```python
from build123d import *

# Parameters (mm, degrees)
BOSS_EXTRUDE4_DEPTH = 21
BOSS_EXTRUDE5_START = 3.5
BOSS_EXTRUDE5_DEPTH = 3.5
SKETCH4_W           = 27
SKETCH4_H           = 19
CUT_EXTRUDE4_DEPTH  = 72.268857154
SKETCH3_5_W         = 24.4
SKETCH3_5_H         = 12.66
BOSS_EXTRUDE6_DEPTH = 2
SKETCH5_W           = 51
SKETCH5_H           = 30
BOSS_EXTRUDE7_DEPTH = 10
CUT_EXTRUDE5_DEPTH  = 75.828136419
CUT_EXTRUDE6_REACH  = 76.828
SKETCH8_W           = 24.5
SKETCH8_H           = 19.5
CHAMFER1_SIZE       = 2


with BuildPart() as part:
    # Sketch3 → Boss-Extrude4 (new body)
    with BuildSketch(Plane(origin=(0, 0, 0), x_dir=(1, 0, 0), z_dir=(0, 1, 0))):
        with BuildLine():
            Line((-27, 15), (-27, -39.5))
            ThreePointArc((-27, -39.5), (-26.414213562, -40.914213562), (-25, -41.5))
            Line((-25, -41.5), (25, -41.5))
            ThreePointArc((25, -41.5), (26.414213562, -40.914213562), (27, -39.5))
            Line((27, -39.5), (27, 15))
            ThreePointArc((27, 15), (26.414213562, 16.414213562), (25, 17))
            Line((25, 17), (-25, 17))
            ThreePointArc((-25, 17), (-26.414213562, 16.414213562), (-27, 15))
        make_face()
    extrude(amount=-BOSS_EXTRUDE4_DEPTH)

    # Sketch3<3> → Boss-Extrude5 (add)
    with BuildSketch(Plane(origin=(0, 0, 0), x_dir=(1, 0, 0), z_dir=(0, 1, 0)).offset(BOSS_EXTRUDE5_START)):
        with BuildLine():
            Line((-27, 15), (-27, -39.5))
            ThreePointArc((-27, -39.5), (-26.414213562, -40.914213562), (-25, -41.5))
            Line((-25, -41.5), (25, -41.5))
            ThreePointArc((25, -41.5), (26.414213562, -40.914213562), (27, -39.5))
            Line((27, -39.5), (27, 15))
            ThreePointArc((27, 15), (26.414213562, 16.414213562), (25, 17))
            Line((25, 17), (-25, 17))
            ThreePointArc((-25, 17), (-26.414213562, 16.414213562), (-27, 15))
        make_face()
        Polygon((0, 12), (-1.1, 12), (-1.1, -3.66), (-25.5, -3.66), (-25.5, 15.5), (25.5, 15.5), (25.5, -0.96), (0, -0.96), align=None, mode=Mode.SUBTRACT)
    extrude(amount=-BOSS_EXTRUDE5_DEPTH)

    # Sketch4 → Cut-Extrude4 (cut, through all)
    with BuildSketch(Plane.ZY.offset(27)):
        with Locations((-1.5, -9.5)):
            Rectangle(SKETCH4_W, SKETCH4_H)
    extrude(amount=-CUT_EXTRUDE4_DEPTH, mode=Mode.SUBTRACT)

    # Sketch3<5> → Boss-Extrude6 (add)
    with BuildSketch(Plane(origin=(0, 0, 0), x_dir=(1, 0, 0), z_dir=(0, 1, 0))):
        with Locations((-13.3, 5.67)):
            Rectangle(SKETCH3_5_W, SKETCH3_5_H)
        Polygon((25.5, 12), (0, 12), (0, -0.96), (25.5, -0.96), (25.5, -0.5), align=None)
    extrude(amount=BOSS_EXTRUDE6_DEPTH)

    # Sketch5 → Boss-Extrude7 (add)
    # profile 1 of 2: a face of its own
    with BuildSketch(Plane.XZ.offset(21)):
        with BuildLine():
            ThreePointArc((25, -17), (26.414213562, -16.414213562), (27, -15))
            Line((27, -15), (27, 39.5))
            ThreePointArc((27, 39.5), (26.414213562, 40.914213562), (25, 41.5))
            Line((25, 41.5), (-25, 41.5))
            ThreePointArc((-25, 41.5), (-26.414213562, 40.914213562), (-27, 39.5))
            Line((-27, 39.5), (-27, -15))
            ThreePointArc((-27, -15), (-26.414213562, -16.414213562), (-25, -17))
            Line((-25, -17), (25, -17))
        make_face()
        with Locations((0, -1.5)):
            Rectangle(SKETCH5_W, SKETCH5_H, mode=Mode.SUBTRACT)
    # profile 2 of 2: a face of its own
    with BuildSketch(Plane.XZ.offset(21)):
        with BuildLine():
            ThreePointArc((25, -17), (26.414213562, -16.414213562), (27, -15))
            Line((27, -15), (27, 39.5))
            ThreePointArc((27, 39.5), (26.414213562, 40.914213562), (25, 41.5))
            Line((25, 41.5), (-25, 41.5))
            ThreePointArc((-25, 41.5), (-26.414213562, 40.914213562), (-27, 39.5))
            Line((-27, 39.5), (-27, -15))
            ThreePointArc((-27, -15), (-26.414213562, -16.414213562), (-25, -17))
            Line((-25, -17), (25, -17))
        make_face()
        with Locations((0, -1.5)):
            Rectangle(SKETCH5_W, SKETCH5_H, mode=Mode.SUBTRACT)
    extrude(amount=BOSS_EXTRUDE7_DEPTH)

    # Sketch6 → Cut-Extrude5 (cut, through all)
    with BuildSketch(Plane.ZY.offset(27)):
        with BuildLine():
            Line((-10.438825699, -23), (8.061174301, -23))
            ThreePointArc((8.061174301, -23), (8.768281082, -23.292893219), (9.061174301, -24))
            Line((9.061174301, -24), (9.061174301, -27))
            ThreePointArc((9.061174301, -27), (8.768281082, -27.707106781), (8.061174301, -28))
            Line((8.061174301, -28), (-10.438825699, -28))
            ThreePointArc((-10.438825699, -28), (-11.14593248, -27.707106781), (-11.438825699, -27))
            Line((-11.438825699, -27), (-11.438825699, -24))
            ThreePointArc((-11.438825699, -24), (-11.14593248, -23.292893219), (-10.438825699, -23))
        make_face()
    extrude(amount=-CUT_EXTRUDE5_DEPTH, mode=Mode.SUBTRACT)

    # Sketch8 → Cut-Extrude6 (cut, up to next)
    with BuildSketch(Plane(origin=(27, 0, 0), x_dir=(0, 0, -1), z_dir=(1, 0, 0)), mode=Mode.PRIVATE) as cut_extrude6_sk1:
        with Locations((-27.25, -9.75)):
            Rectangle(SKETCH8_W, SKETCH8_H)
    cut_extrude6_tool1 = extrude(cut_extrude6_sk1.sketch, amount=-CUT_EXTRUDE6_REACH, mode=Mode.PRIVATE) & part.part
    add(cut_extrude6_tool1.solids().sort_by_distance((27, -9.75, 27.25))[0], mode=Mode.SUBTRACT)

    # Chamfer1
    chamfer1_edges = [part.edges().sort_by_distance(p)[0] for p in [
        (25.5, -26, -16.5),
        (-25.5, -21, -1.5),
        (-25.5, -26, -16.5),
        (0, -21, 13.5),
        (-25.5, -26, 13.5),
        (25.5, -26, 13.5),
        (0, -21, -16.5),
        (25.5, -21, -1.5),
        (0, 0, 12),
        (0, -19, 12),
    ]]
    chamfer(chamfer1_edges, length=CHAMFER1_SIZE - 0.0001)  # a hair under: the kernel refuses the full size


solid = part.part
```
The model under review builds one solid part; all positions refer to its coordinate system, in mm. A direction names the side the tool comes from. Round coordinates to 2 decimals unless told otherwise and drop trailing zeros. Order: outer loops, then holes, each group sorted by start corner. A loop starts at its lowest first (then second) coordinate and runs counter-clockwise, first axis right, second up. Notation, with made-up numbers: (60, 51.5) -> (90, 51.5) arc R21 ccw to (90, 56.5) -> close; hole circle Ø6 at (32, 31.25). An arc over 180 degrees is marked (long way). Use a Markdown table: item, result.
Q1. Tool access review of faces 1 (the flat face through (-26, -28, -1)), 2 (the flat face through (13, 2, -6)), 3 (the flat face through (-25.5, -29, -2)): name each direction out of +Z, -Z, +X, -X, +Y, -Y from which nothing blocks a thin tool from reaching the whole face with its end or side.
Values:
| item | result |
|---|---|
| face 1 | +X, -X |
| face 2 | +Y |
| face 3 | -Y |
Q2. Mouldability with a two-part tool opening along Y and no side actions: class faces 4 (the flat face through (26, -28, -1)), 5 (the flat face through (0, -21, -2)), 6 (the flat face through (-13, 2, 3.66)), 7 (the flat face through (-26, -25, 9.061)) as +Y half, -Y half, draft (parallel to the pull), parting line (faces both ways), or undercut.
Values:
| item | result |
|---|---|
| face 4 | undercut |
| face 5 | -Y half |
| face 6 | draft |
| face 7 | undercut |
Q3. We need section D-D on y = -29. Write out the cut boundary in (x, z).
Values:
| item | result |
|---|---|
| outline | (-27, -15) arc R2 ccw to (-25, -17) -> (25, -17) arc R2 ccw to (27, -15) -> (27, 39.5) arc R2 ccw to (25, 41.5) -> (-25, 41.5) arc R2 ccw to (-27, 39.5) -> close; hole (-25.5, -14.5) -> (-23.5, -16.5) -> (23.5, -16.5) -> (25.5, -14.5) -> (25.5, 11.5) -> (23.5, 13.5) -> (-23.5, 13.5) -> (-25.5, 11.5) -> close |
Q4. We need section B-B on z = 7. State how many separate pieces and enclosed holes the cut face has, then the cut area to 3 significant figures.
Values:
| item | result |
|---|---|
| separate pieces | 4 |
| enclosed holes | 0 |
| area | 316 mm^2 |
Q5. For line 1 (Z direction, x = -9, y = -10); line 2 (Z direction, x = 3, y = -26); line 3 (X direction, y = -22.5, z = -7), list the stretches that pass through material, from the lowest coordinate up.
Values:
| item | result |
|---|---|
| line 1 | z = -17 to -15, 12 to 15, 39.5 to 41.5 |
| line 2 | z = -17 to -16.5, 13.5 to 41.5 |
| line 3 | x = -27 to -25, 25 to 27 |
Q6. We need section C-C on y = -25.5. Write out the cut boundary in (x, z), then the cut area to 3 significant figures.
Values:
| item | result |
|---|---|
| outline | (-27, -15) arc R2 ccw to (-25, -17) -> (25, -17) arc R2 ccw to (27, -15) -> (27, -11.44) -> (25.5, -11.44) -> (25.5, -14.5) -> (23.5, -16.5) -> (-23.5, -16.5) -> (-25.5, -14.5) -> (-25.5, -11.44) -> (-27, -11.44) -> close; (-27, 9.06) -> (-25.5, 9.06) -> (-25.5, 11.5) -> (-23.5, 13.5) -> (23.5, 13.5) -> (25.5, 11.5) -> (25.5, 9.06) -> (27, 9.06) -> (27, 39.5) arc R2 ccw to (25, 41.5) -> (-25, 41.5) arc R2 ccw to (-27, 39.5) -> close |
| area | 1,570 mm^2 |
Q7. Clearance check with flat-ended pins moving along their axes: P1, Ø20, axis at x = -1, z = -1, coming from the -Y side; P2, Ø0.8, axis at x = -26.5, y = -25.5, coming from the -Z side. State where each tip first meets the part, or that it passes through.
Values:
| item | result |
|---|---|
| P1 | stops at y = -21 |
| P2 | stops at z = -16.67 |
Q8. We need section A-A on x = -5. Write out the cut boundary in (y, z), then the cut area to 3 significant figures.
Values:
| item | result |
|---|---|
| outline | (-31, -17) -> (3.5, -17) -> (3.5, -15.5) -> (0, -15.5) -> (0, -15) -> (-19, -15) -> (-19, 10) -> (-17, 12) -> (-2, 12) -> (0, 10) -> (0, 3.66) -> (3.5, 3.66) -> (3.5, 41.5) -> (-31, 41.5) -> (-31, 13.5) -> (-23, 13.5) -> (-21, 11.5) -> (-21, -14.5) -> (-23, -16.5) -> (-31, -16.5) -> close; (0, -12) -> (2, -12) -> (2, 0.66) -> (0, 0.66) -> close; hole (-19.5, 15) -> (0, 15) -> (0, 39.5) -> (-19.5, 39.5) -> close |
| area | 694 mm^2 |
